CAD build for the part. Positions are in the model's coordinates, mm. A direction names the side the tool comes from. Coordinates: 2 decimals unless noted, no trailing zeros. Loops run counter-clockwise (first coordinate to the right, second up) from the corner with the lowest first, then second, coordinate; pieces in that order, holes last. Notation, with made-up numbers: (61, 71.25) -> (80, 71.25) arc R27 cw to (80, 88.25) -> close; hole circle Ø7 at (65, 39). An arc over 180 degrees is marked (long way). Write each question's results on one line, items separated by ' | '.
```python
from build123d import *

# Parameters (mm, degrees)
BOSS_EXTRUDE1_DEPTH                 = 6.35
SKETCH2_R                           = 1.9526
BOSS_EXTRUDE2_DEPTH                 = 3.175
CUT_EXTRUDE1_DEPTH                  = 3.175158
CUT_EXTRUDE1_DIRECTION_2_REACH      = 95.876
CUT_EXTRUDE1_DIRECTION_2_END_RADIUS = 38.494186542
BOSS_EXTRUDE3_DEPTH                 = 12.7
CHAMFER2_SIZE                       = 12.7
F_9_64_0_14063_DIAMETER_HOLE1_D     = 3.572002
CUT_EXTRUDE4_DEPTH                  = 7.112
BOSS_EXTRUDE4_DEPTH                 = 3.175
BOSS_EXTRUDE4_DEPTH_BACK            = 1.5875
SKETCH12_W                          = 3.175
SKETCH12_H                          = 7.112
BOSS_EXTRUDE6_START                 = -89.684533
BOSS_EXTRUDE6_DEPTH                 = 89.684533
FILLET5_R                           = 3.175
SKETCH18_W                          = 83.334533228
SKETCH18_H                          = 26.913353796
CUT_EXTRUDE8_DEPTH                  = 71.073899328
CUT_EXTRUDE6_DEPTH                  = 71.563193649
CUT_EXTRUDE6_DEPTH_BACK             = 71.563193649
SKETCH15_W                          = 3.175
SKETCH15_H                          = 3.175
FILLET6_R                           = 1.5875


with BuildPart() as part:
    # Sketch1 → Boss-Extrude1 (new body)
    with BuildSketch(Plane.XY):
        with BuildLine():
            Line((44.842266614, 13.1), (30.393088537, 28.505811271))
            ThreePointArc((30.393088537, 28.505811271), (0, 41.669186542), (-30.393088537, 28.505811271))
            Line((-30.393088537, 28.505811271), (-44.842266614, 13.1))
            Line((-44.842266614, 13.1), (-44.842266614, 0.4))
            Line((-44.842266614, 0.4), (-41.667266614, 0.4))
            Line((-41.667266614, 0.4), (-38.49210825, 0.4))
            ThreePointArc((-38.49210825, 0.4), (0, 38.494186542), (38.49210825, 0.4))
            Line((38.49210825, 0.4), (41.667266614, 0.4))
            Line((41.667266614, 0.4), (44.842266614, 0.4))
            Line((44.842266614, 0.4), (44.842266614, 13.1))
        make_face()
    extrude(amount=BOSS_EXTRUDE1_DEPTH)

    # Sketch2 → Boss-Extrude2 (add)
    with BuildSketch(Plane(origin=(44.842266614, 0, 0), x_dir=(0, 0, -1), z_dir=(1, 0, 0))):
        with BuildLine():
            Line((0, 13.1), (9.880631277, 3.71845728))
            ThreePointArc((9.880631277, 3.71845728), (10.572747241, -2.908726095), (4.134101417, -4.624075608))
            Line((4.134101417, -4.624075608), (-6.35, 0.4))
            Line((-6.35, 0.4), (0, 0.4))
            Line((0, 0.4), (0, 13.1))
        make_face()
        with Locations((6.35, 0)):
            Circle(SKETCH2_R, mode=Mode.SUBTRACT)
    boss_extrude2 = extrude(amount=-BOSS_EXTRUDE2_DEPTH)

    # Mirror1: Boss-Extrude2 across plane
    add(boss_extrude2.mirror(Plane(origin=(0, 0, 0), x_dir=(0, 0, 1), z_dir=(1, 0, 0))))

    # Sketch4 → Cut-Extrude1 (cut)
    with BuildSketch(Plane(origin=(-38.49210825, 0, 0), x_dir=(0, 0, -1), z_dir=(1, 0, 0))):
        Polygon((-6.35, 0.4), (0, 3.194), (0, 0.4), align=None)
    extrude(amount=-CUT_EXTRUDE1_DEPTH, mode=Mode.SUBTRACT)

    # Cut-Extrude1 direction 2: up to this cylinder (the profile starts outside it)
    cut_extrude1_direction_2_end = Plane(origin=(0, 0, 2.116667), z_dir=(0, 0, -1)) * Cylinder(CUT_EXTRUDE1_DIRECTION_2_END_RADIUS, 269.740373084, mode=Mode.PRIVATE)
    # Sketch4 → Cut-Extrude1 direction 2 (cut, up to the surface)
    with BuildSketch(Plane(origin=(-38.49210825, 0, 0), x_dir=(0, 0, -1), z_dir=(1, 0, 0)), mode=Mode.PRIVATE) as cut_extrude1_direction_2_sk1:
        Polygon((-6.35, 0.4), (0, 3.194), (0, 0.4), align=None)
    cut_extrude1_direction_2_tool1 = extrude(cut_extrude1_direction_2_sk1.sketch, amount=CUT_EXTRUDE1_DIRECTION_2_REACH, mode=Mode.PRIVATE) - cut_extrude1_direction_2_end
    add(cut_extrude1_direction_2_tool1.solids().sort_by_distance((-38.492108, 1.331333, 2.116667))[0], mode=Mode.SUBTRACT)

    # Sketch5 → Boss-Extrude3 (add)
    with BuildSketch(Plane.XY.offset(6.35)):
        with BuildLine():
            Line((-6.35, 38.374458705), (-6.35, 41.182503652))
            ThreePointArc((-6.35, 41.182503652), (0, 41.669186542), (6.35, 41.182503652))
            Line((6.35, 41.182503652), (6.35, 38.374458705))
            Line((6.35, 38.374458705), (5.95, 38.43637921))
            ThreePointArc((5.95, 38.43637921), (0, 38.894186542), (-5.95, 38.43637921))
            Line((-5.95, 38.43637921), (-6.35, 38.374458705))
        make_face()
    extrude(amount=BOSS_EXTRUDE3_DEPTH)

    # Chamfer2
    # the kernel refuses this chamfer: 12.7 mm, written as the material it adds along each edge
    with BuildSketch(Plane(origin=(6.35, 73.842877599, 6.35), x_dir=(0.9996219169112968, 0, -0.02749587661058633), z_dir=(0, -1, 0))) as chamfer2_piece_1_section:
        Polygon((CHAMFER2_SIZE * 0.999621916911, CHAMFER2_SIZE * 0.0274958766106), (-CHAMFER2_SIZE * 0.0274958766106, CHAMFER2_SIZE * 0.999621916911), (0, 0), align=None)
    chamfer2_piece_1 = extrude(amount=68.128792841, mode=Mode.PRIVATE)
    chamfer2_piece_1 = chamfer2_piece_1 & Plane(origin=(0, 0, 10.815604597), x_dir=(0.7293900135753609, 0.6840980982991656, 0), z_dir=(0, 0, -1)) * Cylinder(41.669186542, 188, mode=Mode.PRIVATE)
    chamfer2_piece_1 = split(chamfer2_piece_1, bisect_by=Plane(origin=(9.796586026, 37.840922839, 10.815604597), z_dir=(0.15297916035843936, 0.988229414911349, 0)), keep=Keep.TOP, mode=Mode.PRIVATE)
    chamfer2_piece_1 = split(chamfer2_piece_1, bisect_by=Plane(origin=(9.988062905, 39.077843499, 19.05), z_dir=(0, 0, -1)), keep=Keep.TOP, mode=Mode.PRIVATE)
    add(chamfer2_piece_1)
    with BuildSketch(Plane(origin=(-6.35, 5.714084758, 6.35), x_dir=(-0.9996219169112966, 0, -0.0274958766105864), z_dir=(0, 1, 0))) as chamfer2_piece_2_section:
        Polygon((CHAMFER2_SIZE * 0.999621916911, CHAMFER2_SIZE * 0.0274958766106), (-CHAMFER2_SIZE * 0.0274958766106, CHAMFER2_SIZE * 0.999621916911), (0, 0), align=None)
    chamfer2_piece_2 = extrude(amount=68.128792841, mode=Mode.PRIVATE)
    chamfer2_piece_2 = chamfer2_piece_2 & Plane(origin=(0, 0, 10.81560458), x_dir=(0.7293900135753609, 0.6840980982991656, 0), z_dir=(0, 0, -1)) * Cylinder(41.669186542, 188, mode=Mode.PRIVATE)
    chamfer2_piece_2 = split(chamfer2_piece_2, bisect_by=Plane(origin=(-9.796586033, 37.840922838, 10.81560458), z_dir=(-0.15297916035843936, 0.988229414911349, 0)), keep=Keep.TOP, mode=Mode.PRIVATE)
    chamfer2_piece_2 = split(chamfer2_piece_2, bisect_by=Plane(origin=(-9.988062912, 39.077843496, 19.05), z_dir=(0, 0, -1)), keep=Keep.TOP, mode=Mode.PRIVATE)
    add(chamfer2_piece_2)

    # 9/64 (0.14063) Diameter Hole1 (through all)
    with Locations(Plane(origin=(0, 41.669186542, 0), x_dir=(1, 0, 0), z_dir=(0, 1, 0))):
        with Locations((0, -3.44678)):
            Hole(F_9_64_0_14063_DIAMETER_HOLE1_D / 2)

    # Sketch11 → Cut-Extrude4 (cut)
    with BuildSketch(Plane(origin=(0, 0, 0), x_dir=(-1, 0, 0), z_dir=(0, 0, -1))):
        with BuildLine():
            ThreePointArc((6.35, 41.182503652), (0, 41.669186542), (-6.35, 41.182503652))
            Line((-6.35, 41.182503652), (6.35, 41.182503652))
        make_face()
    extrude(amount=-CUT_EXTRUDE4_DEPTH, mode=Mode.SUBTRACT)

    # Sketch12 → Boss-Extrude4 (add, two sides: drawn at the far end of the back side and taken through both)
    with BuildSketch(Plane(origin=(0, 41.182503652, 0), x_dir=(1, 0, 0), z_dir=(0, 1, 0)).offset(-BOSS_EXTRUDE4_DEPTH_BACK)):
        with Locations((-5.0355, -3.556)):
            Rectangle(SKETCH12_W, SKETCH12_H)
        with Locations((5.0355, -3.556)):
            Rectangle(SKETCH12_W, SKETCH12_H)
    extrude(amount=BOSS_EXTRUDE4_DEPTH + BOSS_EXTRUDE4_DEPTH_BACK)

    # Sketch16 → Boss-Extrude6 (add)
    with BuildSketch(Plane(origin=(44.842266614, 0, 0), x_dir=(0, 0, -1), z_dir=(1, 0, 0)).offset(BOSS_EXTRUDE6_START)):
        with BuildLine():
            Line((-1.107949291, -2.112037804), (5.579304246, -14.434735992))
            Line((5.579304246, -14.434735992), (0, -17.4625))
            Line((0, -17.4625), (0, -20.6375))
            Line((0, -20.6375), (9.8901, -20.6375))
            ThreePointArc((9.8901, -20.6375), (11.012632015, -20.172532015), (11.4776, -19.05))
            Line((11.4776, -19.05), (11.4776, 0))
            ThreePointArc((11.4776, 0), (9.082218896, -4.339039256), (4.134101417, -4.624075608))
            Line((4.134101417, -4.624075608), (-1.107949291, -2.112037804))
        make_face()
    boss_extrude6 = extrude(amount=BOSS_EXTRUDE6_DEPTH)

    # Fillet5
    fillet5_edges = [part.edges().sort_by_distance(p)[0] for p in [
        (43.254766614, -2.112037804, 1.107949291),
    ]]
    fillet(fillet5_edges, radius=FILLET5_R)

    # Mirror4: Boss-Extrude6 across plane
    add(boss_extrude6.mirror(Plane(origin=(0, 0, 0), x_dir=(0, 0, 1), z_dir=(1, 0, 0))))

    # Sketch18 → Cut-Extrude8 (cut, through all)
    with BuildSketch(Plane(origin=(0, 0, -11.4776), x_dir=(-1, 0, 0), z_dir=(0, 0, -1))):
        with Locations((0, -13.456676898)):
            Rectangle(SKETCH18_W, SKETCH18_H)
    extrude(amount=-CUT_EXTRUDE8_DEPTH, mode=Mode.SUBTRACT)

    # Sketch15 → Cut-Extrude6 (cut, two sides: drawn at the far end of the back side and taken through both)
    with BuildSketch(Plane(origin=(6.623, 0, 0), x_dir=(0, 0, -1), z_dir=(1, 0, 0)).offset(-CUT_EXTRUDE6_DEPTH_BACK)):
        with Locations((-1.5875, 42.770003652)):
            Rectangle(SKETCH15_W, SKETCH15_H)
    extrude(amount=CUT_EXTRUDE6_DEPTH + CUT_EXTRUDE6_DEPTH_BACK, mode=Mode.SUBTRACT)

    # Fillet6
    fillet6_edges = [part.edges().sort_by_distance(p)[0] for p in [
        (-43.2547665, -20.6375, 0),
        (-43.2547665, -17.4625, 0),
        (-43.2547665, -14.434735992, -5.579304246),
        (43.254766614, -14.434735992, -5.579304246),
        (43.254766614, -17.4625, 0),
        (43.254766614, -20.6375, 0),
    ]]
    fillet(fillet6_edges, radius=FILLET6_R)


solid = part.part
```
Q1. Cut at A-A on x = 0. Write the cut outline in (y, z).
Results are:
outline: (38.49, 0) -> (41.18, 0) -> (41.18, 1.66) -> (38.49, 1.66) -> close; (38.49, 5.23) -> (41.18, 5.23) -> (41.18, 7.11) -> (41.67, 7.11) -> (41.67, 19.05) -> (38.89, 19.05) -> (38.89, 6.35) -> (38.49, 6.35) -> close
Q2. Cut at B-B on y = 11. Write the cut outline in (x, z).
Results are:
outline: (-44.84, -2.21) -> (-41.67, -2.21) -> (-41.67, 0) -> (-36.89, 0) -> (-36.89, 6.35) -> (-44.84, 6.35) -> close; (36.89, 0) -> (41.67, 0) -> (41.67, -2.21) -> (44.84, -2.21) -> (44.84, 6.35) -> (36.89, 6.35) -> close
Q3. Cut at C-C on z = -6.35. Write the cut outline in (x, y).
Results are:
outline: (-44.84, -20.64) -> (-41.67, -20.64) -> (-41.67, -1.95) -> (-44.84, -1.95) -> close; (-44.84, 1.95) -> (-41.67, 1.95) -> (-41.67, 7.07) -> (-44.84, 7.07) -> close; (41.67, -20.64) -> (44.84, -20.64) -> (44.84, -1.95) -> (41.67, -1.95) -> close; (41.67, 1.95) -> (44.84, 1.95) -> (44.84, 7.07) -> (41.67, 7.07) -> close
Q4. Drop flat-ended pins along their axis: pin 1 (1 mm diameter, centred on x = 5, y = 42, fed in from -Z) (3 decimals); pin 2 (0.5 mm diameter, centred on x = -43.5, y = -19, fed in from +Z); pin 3 (4 mm diameter, centred on x = -35.5, z = 5.5, fed in from +Y); pin 4 (10 mm diameter, centred on x = 14.5, y = 27, fed in from +Z). Give the stop position or say it passes through.
Results are:
pin 1: z = 3.175 | pin 2: z = 0 | pin 3: y = 25.19 | pin 4: through
Q5. Cut at D-D on y = 40. Write the cut outline in (x, z).
Results are:
outline: (-11.68, 0) -> (11.68, 0) -> (11.68, 13.72) -> (6.35, 19.05) -> (-6.35, 19.05) -> (-11.68, 13.72) -> close; hole circle Ø3.57 at (0, 3.45)
Q6. Pull direction Y, two halves, no side cores. Call faces 5 (the flat face through (-43.28, -16.09, -2.53)), 6 (the flat face through (40, 0.4, 3)), 7 (the flat face through (-3.448, 43, 5)): +Y half, -Y half, draft (parallel to the pull), parting line (faces both ways), or undercut.
Results are:
face 5: undercut | face 6: -Y half | face 7: draft
Q7. Which spindle directions (+Z, -Z, +X, -X, +Y, -Y) get a long thin tool onto all of the face, cutting with end or side? Do faces 1 (the flat face through (-5, 43, 7.112)), 2 (the flat face through (-6.623, 43, 5)), 3 (the flat face through (43.233, -7.958, -2.064)), 4 (the flat face through (-43, -10, -11.478)). Say none if no direction does.
Results are:
face 1: +Z, -X, +Y | face 2: +Z, -Z, -X, +Y | face 3: +Z, +X, -X | face 4: -Z, +X, -X, +Y, -Y
Q8. Wall check: L1, parallel to Z at x = 0, y = 40; L2, parallel to X at y = 9, z = -3.5; L3, parallel to Y at x = 43.35, z = -6.35. Give the ranges that are in metal, low to high. Write a range as from..to.
Results are:
L1: 0..1.66, 5.23..19.05 | L2: -44.84..-41.67, 41.67..44.84 | L3: -20.64..-1.95, 1.95..7.07
